Input: dimensioned drawing with shaded views. Units: mm. Origin: part minimum x, y, z. Round coordinates to 2 decimals unless told otherwise and drop trailing zeros. Loops run counter-clockwise (first coordinate to the right, second up) from the corner with the lowest first, then second, coordinate; pieces in that order, holes last. Notation, with made-up numbers: M -29.75,26.25 L -19.75,26.25 A17 ccw -19.75,46.25 Z; hole C 19.25,58 d2. An arc over 180 degrees is marked long. Write each question's results on one line, items separated by ' | '. Start each with the question number.
1. Section D-D on y = 0.7. Output: boundary loops of the cut face in (x, z).
2. Section A-A on z = 11. Output: boundary loops of the cut face in (x, y), and give its area (3 significant figures).
3. Section B-B on x = 61. Output: boundary loops of the cut face in (y, z), and give its area (3 significant figures).
4. Contact query for flat-ended pins moving along their axis: pin 1 Ø1.5 at (x, y) = (11.5, 0.5) entering from -Z; pin 2 Ø1.5 at (x, y) = (57, 1.5) entering from +Z. Output: stop coordinate, or through.
5. Ray query, line 1 (X direction, y = 0.9, z = 52); line 2 (Z direction, x = 3, y = 2.1); line 3 (Z direction, x = 23.5, y = 0.1). Return the intervals inside material, ascending.
6. Draft query along Y for the marked faces 1 and 2. Return one class per face: released by +Y, released by -Y, zero draft, split by the parting line, or undercut.
7. Section C-C on x = 36. Output: boundary loops of the cut face in (y, z).
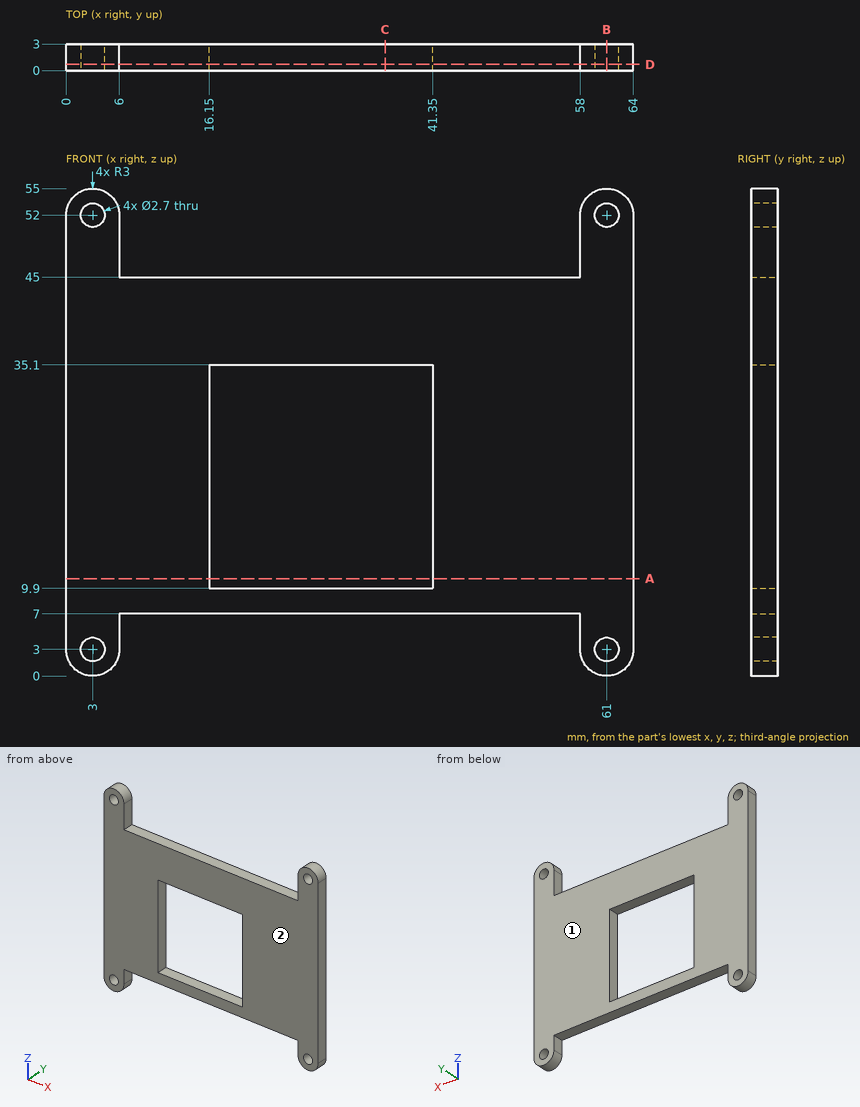
Taken from the geometry:
1) outline: M 0,3 A3 ccw 6,3 L 6,7 L 58,7 L 58,3 A3 ccw 64,3 L 64,52 A3 ccw 58,52 L 58,45 L 6,45 L 6,52 A3 ccw 0,52 Z; hole C 3,3 d2.7; hole C 3,52 d2.7; hole M 16.15,9.9 L 41.35,9.9 L 41.35,35.1 L 16.15,35.1 Z; hole C 61,3 d2.7; hole C 61,52 d2.7
2) outline: M 0,0 L 16.15,0 L 16.15,3 L 0,3 Z; M 41.35,0 L 64,0 L 64,3 L 41.35,3 Z | area: 116 mm^2
3) outline: M 0,0 L 3,0 L 3,1.65 L 0,1.65 Z; M 0,4.35 L 3,4.35 L 3,50.65 L 0,50.65 Z; M 0,53.35 L 3,53.35 L 3,55 L 0,55 Z | area: 149 mm^2
4) pin 1: z = 7 | pin 2: z = 45
5) line 1: 0 to 1.65, 4.35 to 6, 58 to 59.65, 62.35 to 64 | line 2: 0 to 1.65, 4.35 to 50.65, 53.35 to 55 | line 3: 7 to 9.9, 35.1 to 45
6) face 1: released by +Y | face 2: released by -Y
7) outline: M 0,7 L 3,7 L 3,9.9 L 0,9.9 Z; M 0,35.1 L 3,35.1 L 3,45 L 0,45 Z
